```python
from build123d import *

# Parameters (mm, degrees)
BOSS_EXTRUDE1_DEPTH = 7.25
CUT_EXTRUDE1_DEPTH  = 50
CUT_EXTRUDE2_DEPTH  = 50
SKETCH2_4_R         = 2.125
CUT_EXTRUDE3_DEPTH  = 50
SKETCH6_R           = 2.125
CUT_EXTRUDE4_DEPTH  = 50


with BuildPart() as part:
    # Sketch1 → Boss-Extrude1 (new body)
    with BuildSketch(Plane.XY):
        with BuildLine():
            Line((0, 0), (0, 12.55))
            ThreePointArc((0, 12.55), (0.366116524, 13.433883476), (1.25, 13.8))
            Line((1.25, 13.8), (10.25, 13.8))
            ThreePointArc((10.25, 13.8), (11.133883476, 13.433883476), (11.5, 12.55))
            Line((11.5, 12.55), (11.5, 0))
            Line((11.5, 0), (10.75, 0))
            Line((10.75, 0), (10.75, 13.05))
            Line((10.75, 13.05), (0.75, 13.05))
            Line((0.75, 13.05), (0.75, 0))
            Line((0.75, 0), (0, 0))
        make_face()
    extrude(amount=BOSS_EXTRUDE1_DEPTH)

    # Sketch2 → Cut-Extrude1 (cut, symmetric)
    with BuildSketch(Plane.ZY):
        with BuildLine():
            Line((0, 0), (3.625, 0))
            ThreePointArc((3.625, 0), (1.061737918, 1.061737918), (0, 3.625))
            Line((0, 3.625), (0, 0))
        make_face()
    extrude(amount=CUT_EXTRUDE1_DEPTH, both=True, mode=Mode.SUBTRACT)

    # Sketch2<3> → Cut-Extrude2 (cut, symmetric)
    with BuildSketch(Plane.ZY):
        with BuildLine():
            ThreePointArc((7.25, 3.625), (6.188262082, 1.061737918), (3.625, 0))
            Line((3.625, 0), (7.25, 0))
            Line((7.25, 0), (7.25, 3.625))
        make_face()
    extrude(amount=CUT_EXTRUDE2_DEPTH, both=True, mode=Mode.SUBTRACT)

    # Sketch2<4> → Cut-Extrude3 (cut, symmetric)
    with BuildSketch(Plane.ZY):
        with Locations((3.625, 3.625)):
            Circle(SKETCH2_4_R)
    extrude(amount=CUT_EXTRUDE3_DEPTH, both=True, mode=Mode.SUBTRACT)

    # Sketch6 → Cut-Extrude4 (cut, symmetric)
    with BuildSketch(Plane(origin=(0, 13.8, 0), x_dir=(1, 0, 0), z_dir=(0, 1, 0))):
        with Locations((5.75, -3.625)):
            Circle(SKETCH6_R)
    extrude(amount=CUT_EXTRUDE4_DEPTH, both=True, mode=Mode.SUBTRACT)


solid = part.part
```
Check sheet for the modelled part. Datum: model origin and axes. Units: mm. A direction names the side the tool comes from. Coordinates: 2 decimals unless noted, no trailing zeros. Write each loop counter-clockwise with the first axis right and the second up, starting at its lowest first coordinate (ties: lowest second). Pieces come first, ordered by that corner, then holes. Notation, with made-up numbers: M 61.25,-18.75 L 114.25,-18.75 A26 ccw 114.25,6.25 Z; hole C 20,70 d9. An arc over 180 degrees is marked long. Write item = value, one per line. Start each with the question number.
1. Sectioned sample at B-B (x = 5.75). Record the cut outline in (y, z), then the cut area to 3 significant figures.
2. Thickness scan on probe 1 along X at (y, z) = (10.25, 1.5); probe 2 along Y at (x, z) = (6.75, 6.5); probe 3 along X at (y, z) = (13, 2.5). Record the ranges inside material, lowest first.
3. Mould release check, pull along Z, two halves, no side actions. Record for faces 3 (the flat face through (5.8, 13.3, 7.25)), 4 (the cylindrical face through (5.3, 13.4, 5.7)), 5 (the flat face through (11.5, 8, 4)), 6 (the flat face through (5.8, 13.3, 0)): pulls with the +Z half, pulls with the -Z half, needs draft (parallel to the pull), parting line crosses it, or undercut.
4. Sectioned sample at A-A (y = 11.75). Record the cut outline in (x, z).
5. Sectioned sample at C-C (z = 4). Record the cut outline in (x, y), then the cut area to 3 significant figures.
6. Tool access check on faces 1 (the flat face through (0.75, 8, 4)), 2 (the cylindrical face through (11.124, 13.444, 3.574)). Record the directions out of +Z, -Z, +X, -X, +Y, -Y that give a thin tool (end or side, any length) a straight path to the whole face; none if there is none.
7. Sectioned sample at D-D (y = 5.5). Record the cut outline in (x, z) (3 decimals).
The answers:
q1.outline = M 13.05,0 L 13.8,0 L 13.8,1.5 L 13.05,1.5 Z; M 13.05,5.75 L 13.8,5.75 L 13.8,7.25 L 13.05,7.25 Z
q1.area = 2.25 mm²
q2.probe_1 = 0 to 0.75, 10.75 to 11.5
q2.probe_2 = 13.05 to 13.8
q2.probe_3 = 0.08 to 0.75, 10.75 to 11.42
q3.face_3 = pulls with the +Z half
q3.face_4 = undercut
q3.face_5 = needs draft
q3.face_6 = pulls with the -Z half
q4.outline = M 0,0 L 0.75,0 L 0.75,7.25 L 0,7.25 Z; M 10.75,0 L 11.5,0 L 11.5,7.25 L 10.75,7.25 Z
q5.outline = M 0,0.02 L 0.75,0.02 L 0.75,1.53 L 0,1.53 Z; M 0,5.72 L 0.75,5.72 L 0.75,13.05 L 3.66,13.05 L 3.66,13.8 L 1.25,13.8 A1.25 ccw 0,12.55 Z; M 7.84,13.05 L 10.75,13.05 L 10.75,5.72 L 11.5,5.72 L 11.5,12.55 A1.25 ccw 10.25,13.8 L 7.84,13.8 Z; M 10.75,0.02 L 11.5,0.02 L 11.5,1.53 L 10.75,1.53 Z
q5.area = 18.1 mm²
q6.face_1 = +Z, -Z, -Y
q6.face_2 = +Z, -Z, +X, +Y
q7.outline = M 0,0 L 0.75,0 L 0.75,2.625 L 0,2.625 Z; M 0,4.625 L 0.75,4.625 L 0.75,7.25 L 0,7.25 Z; M 10.75,0 L 11.5,0 L 11.5,2.625 L 10.75,2.625 Z; M 10.75,4.625 L 11.5,4.625 L 11.5,7.25 L 10.75,7.25 Z
